Input: part model. Units: mm. Frame: model coordinates. A direction names the side the tool comes from. Give positions to 0.01 mm unless a question says otherwise; leave off trailing zeros. Order: outer loops, then holes, each group sorted by start corner. A loop starts at its lowest first (then second) coordinate and runs counter-clockwise, first axis right, second up.
```python
from build123d import *

# Parameters (mm, degrees)
SKETCH1_R           = 2.5
BOSS_EXTRUDE1_DEPTH = 22
SKETCH3_W           = 2
SKETCH3_H           = 20
CUT_EXTRUDE1_DEPTH  = 15


with BuildPart() as part:
    # Sketch1 → Boss-Extrude1 (new body)
    with BuildSketch(Plane.XY):
        with BuildLine():
            Line((-27.5, 4.630713194), (12.5, 4.630713194))
            Line((12.5, 4.630713194), (12.5, 7.630713194))
            Line((12.5, 7.630713194), (0, 7.630713194))
            ThreePointArc((0, 7.630713194), (-1.767766953, 8.362946241), (-2.5, 10.130713194))
            ThreePointArc((-2.5, 10.130713194), (-7.5, 15.130713194), (-12.5, 10.130713194))
            ThreePointArc((-12.5, 10.130713194), (-13.232233047, 8.362946241), (-15, 7.630713194))
            Line((-15, 7.630713194), (-27.5, 7.630713194))
            Line((-27.5, 7.630713194), (-27.5, 4.630713194))
        make_face()
        with Locations((-7.5, 10.130713194)):
            Circle(SKETCH1_R, mode=Mode.SUBTRACT)
    extrude(amount=BOSS_EXTRUDE1_DEPTH)

    # Sketch3 → Cut-Extrude1 (cut)
    with BuildSketch(Plane(origin=(0, 7.630713194, 0), x_dir=(1, 0, 0), z_dir=(0, 1, 0))):
        with Locations((-25.5, -11)):
            Rectangle(SKETCH3_W, SKETCH3_H)
        with Locations((10.5, -11)):
            Rectangle(SKETCH3_W, SKETCH3_H)
    extrude(amount=-CUT_EXTRUDE1_DEPTH, mode=Mode.SUBTRACT)


solid = part.part
```
1) Cut plane C-C (y = 6). Return the cut outline in (x, z).
2) Cut plane D-D (y = 9.75). Return the cut outline in (x, z), then the cut area to 3 significant figures.
3) Cut plane A-A (z = 8). Return the cut outline in (x, y), then the cut area to 3 significant figures.
4) Pull-direction query (X, two-part tool) for faces 6 (the face through (-24.5, 6, 11)), 7 (the face through (-13.213, 8.382, 10.846)), 8 (the face through (-8, 4.631, 11)); classes: pulls with the +X half, pulls with the -X half, needs draft (parallel to the pull), parting line crosses it, or undercut.
5) Line query: probe 1 along X at (y, z) = (6, 11.75); probe 2 along Y at (x, z) = (-7.5, 6.5); probe 3 along X at (y, z) = (10, 5.75). Output: solid intervals per line, ascending.
6) Reachability of faces 1 (the face through (-21, 7.631, 11)), 2 (the face through (11.5, 6, 11)), 3 (the face through (-7.39, 15.13, 10.85)), 4 (the face through (6, 7.631, 11)), 5 (the face through (-27.5, 6, 11)) from +Z, -Z, +X, -X, +Y, -Y: full face, straight path, thin tool, end or side. Return the list, or none.
7) First-contact query: P1, Ø1.5, axis at y = 11.5, z = 2.5, coming from the +X side; P2, Ø6, axis at x = -19.5, z = 8.5, coming from the +Y side; P3, Ø1.5, axis at x = -0.5, z = 18, coming from the +Y side. Flat tips, straight axial feed; report the tip coordinate or a pass-through.
8) Cut plane B-B (x = -7.5). Return the cut outline in (y, z), then the cut area to 3 significant figures.
Geometry says:
1. outline: (-27.5, 0) - (12.5, 0) - (12.5, 22) - (-27.5, 22) - close; hole (-26.5, 1) - (-24.5, 1) - (-24.5, 21) - (-26.5, 21) - close; hole (9.5, 1) - (11.5, 1) - (11.5, 21) - (9.5, 21) - close
2. outline: (-12.53, 0) - (-9.97, 0) - (-9.97, 22) - (-12.53, 22) - close; (-5.03, 0) - (-2.47, 0) - (-2.47, 22) - (-5.03, 22) - close
2. area: 113 mm2
3. outline: (-27.5, 4.63) - (-26.5, 4.63) - (-26.5, 7.63) - (-27.5, 7.63) - close; (-24.5, 4.63) - (9.5, 4.63) - (9.5, 7.63) - (0, 7.63) arc R2.5 cw to (-2.5, 10.13) arc R5 ccw to (-12.5, 10.13) arc R2.5 cw to (-15, 7.63) - (-24.5, 7.63) - close; (11.5, 4.63) - (12.5, 4.63) - (12.5, 7.63) - (11.5, 7.63) - close; hole circle Ø5 at (-7.5, 10.13)
3. area: 155 mm2
4. face 6: undercut
4. face 7: pulls with the -X half
4. face 8: needs draft
5. probe 1: x = -27.5 to -26.5, -24.5 to 9.5, 11.5 to 12.5
5. probe 2: y = 4.63 to 7.63, 12.63 to 15.13
5. probe 3: x = -12.5 to -10, -5 to -2.5
6. face 1: +Z, -Z, -X, +Y
6. face 2: +Y, -Y
6. face 3: +Z, -Z, +Y
6. face 4: +Z, -Z, +X, +Y
6. face 5: +Z, -Z, -X, +Y, -Y
7. P1: stops at x = -2.54
7. P2: stops at y = 7.63
7. P3: stops at y = 7.97
8. outline: (4.63, 0) - (7.63, 0) - (7.63, 22) - (4.63, 22) - close; (12.63, 0) - (15.13, 0) - (15.13, 22) - (12.63, 22) - close
8. area: 121 mm2
